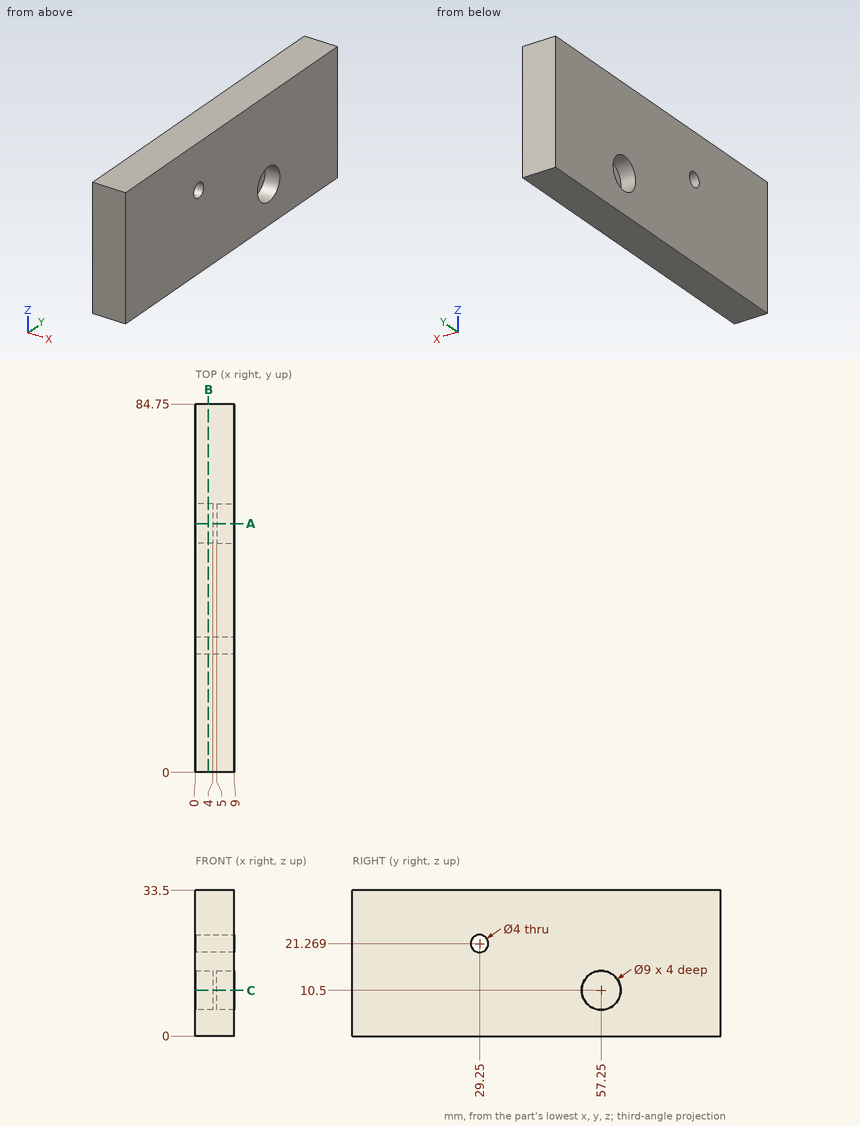
Print and shaded views of the part. All mm, measured from the part's lowest x, y and z. Coordinates: 2 decimals unless noted, no trailing zeros. Order: outer loops, then holes, each group sorted by start corner. A loop starts at its lowest first (then second) coordinate and runs counter-clockwise, first axis right, second up. Notation, with made-up numbers: (70.5, 11) - (97.5, 11) arc R33 ccw to (97.5, 43) - close; hole circle Ø2 at (3.5, 11). An arc over 180 degrees is marked (long way). Put each result on its own line as item: value.
1. Saw through at C-C (z = 10.5). Write the cut outline in (x, y), and give its area (3 significant figures).
Answer sheet:
outline: (0, 0) - (9, 0) - (9, 52.75) - (5, 52.75) - (5, 61.75) - (9, 61.75) - (9, 84.75) - (0, 84.75) - (0, 61.75) - (4, 61.75) - (4, 52.75) - (0, 52.75) - close
area: 691 mm^2
2. Saw through at A-A (y = 57.25). Write the cut outline in (x, z).
Answer sheet:
outline: (0, 0) - (9, 0) - (9, 6) - (5, 6) - (5, 15) - (9, 15) - (9, 33.5) - (0, 33.5) - (0, 15) - (4, 15) - (4, 6) - (0, 6) - close
3. Saw through at B-B (x = 3). Write the cut outline in (y, z), and give its area (3 significant figures).
Answer sheet:
outline: (0, 0) - (84.75, 0) - (84.75, 33.5) - (0, 33.5) - close; hole circle Ø4 at (29.25, 21.27); hole circle Ø9 at (57.25, 10.5)
area: 2,760 mm^2
4. Probe line 1 along Z through (x, y) = (7, 57); line 2 along Y through (x, z) = (7.95, 10.5); line 3 along Z through (x, y) = (3.25, 55.5) (1 decimal). List the from-to ranges inside material, lowest first. Write a range as [from, to].
Answer sheet:
line 1: z = [0, 6.01], [14.99, 33.5]
line 2: y = [0, 52.75], [61.75, 84.75]
line 3: z = [0, 6.4], [14.6, 33.5]
5. Drop flat-ended pins along their axis: P1, Ø7, axis at y = 57.5, z = 10.5, coming from the +X side; P2, Ø4.5, axis at y = 59.5, z = 9, coming from the -X side. Give the stop position or say it passes through.
Answer sheet:
P1: stops at x = 5
P2: stops at x = 0
